Could you check a few things on this model? Use its own coordinates, in mm. Face numbers are marked on the shaded views. A direction names the side the tool comes from. Give positions to 0.01 mm unless a question says otherwise; leave off trailing zeros. Loops run counter-clockwise (first coordinate to the right, second up) from the corner with the lowest first, then second, coordinate; pieces in that order, holes last. Notation, with made-up numbers: (-23.75, 15.25) - (1.25, 15.25) arc R26 cw to (1.25, 35.25) - close; hole circle Ø8 at (13, 47.25). An arc over 180 degrees is marked (long way). Write each question's results on one line, items separated by ' | '. Start each with the question number.
1) I want a section at B-B, the plane x = -5. Write out the boundary of the cut face in (y, z), and give its area (3 significant figures).
2) I want a section at C-C, the plane z = 2.25. Write out the boundary of the cut face in (x, y).
3) I want a section at D-D, the plane y = -4.25. Write out the boundary of the cut face in (x, z).
4) I'm going to push flat-ended pins straight in: pin 1 (3.5 mm diameter, centred on x = -8, y = -2, fed in from +Z); pin 2 (1.8 mm diameter, centred on y = -5.5, z = 2.5, fed in from +X); pin 3 (0.7 mm diameter, centred on x = -8, z = 1.5, fed in from +Y); pin 4 (1.1 mm diameter, centred on x = -7.5, z = 1.5, fed in from -Y). Where does each tip first touch, or does it pass through?
5) On a 3-axis mill with a long thin cutter (end or side, diameter ignored), from which of +Z, -Z, +X, -X, +Y, -Y can I reach the whole of each face in a straight line? I mean the marked faces 1, 2 and 3. Say none if no direction works.
6) If I drill on probe 1 along Y at (x, z) = (-0.25, 4); probe 2 along Y at (x, z) = (-9, 1.25); probe 3 along Z at (x, y) = (10, 1.5), over which ranges is the centre line in solid material (lowest first)? Write a range as [from, to].
7) I want a section at A-A, the plane y = 0. Write out the boundary of the cut face in (x, z).
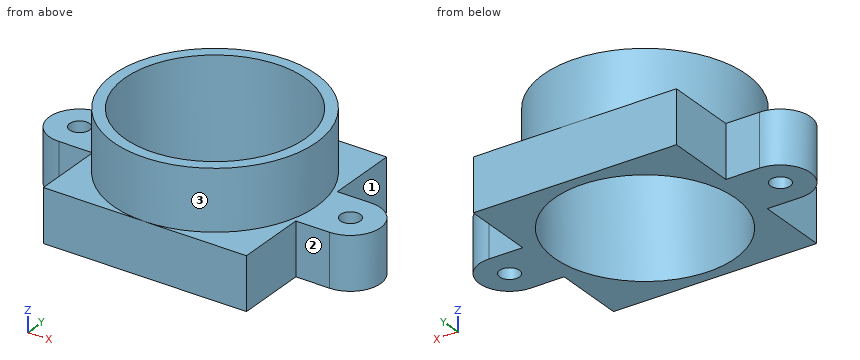
Autodesk Inventor part; units mm, degrees
ref_plane "YZ Plane" through (0, 0, 0) normal (1, 0, 0) x (0, 1, 0)
ref_plane "XZ Plane" through (0, 0, 0) normal (0, 1, 0) x (-1, 0, 0)
ref_plane "XY Plane" through (0, 0, 0) normal (0, 0, 1) x (1, 0, 0)
sketch "Skizze1" plane through (0, 0, 0) normal (0, 0, 1) x (1, 0, 0)
  line L0 (-6.75, -6.75) -> (6.75, -6.75)
  line L1 (6.75, 6.75) -> (-6.75, 6.75)
  line L2 (-6.75, -6.75) -> (6.75, 6.75) construction
  line L3 (6.75, -6.75) -> (-6.75, 6.75) construction
  line L4 (-6.75, 2) -> (-9, 2)
  line L5 (-9, -2) -> (-6.75, -2)
  line L6 (6.75, 2) -> (9, 2)
  line L7 (9, -2) -> (6.75, -2)
  arc A0 (-9, 2) -> (-9, -2) centre (-9, 0) ccw
  arc A1 (9, -2) -> (9, 2) centre (9, 0) ccw
  line L8 (-6.75, 6.75) -> (-6.75, 2)
  line L9 (-6.75, -2) -> (-6.75, -6.75)
  line L10 (6.75, -6.75) -> (6.75, -2)
  line L11 (6.75, 2) -> (6.75, 6.75)
  line L12 (0, 9.45) -> (0, -9.45)
  line L13 (-15.4, 0) -> (15.4, 0)
  point P0 (0, 0)
  dimension "d0" = 13.5
  dimension "d1" = 13.5
  dimension "d2" = 18
  dimension "d3" = 4
extrude "Extrusion1" add sketch "Skizze1" along normal blind 3.5
sketch "Skizze4" plane through (0, 0, 3.5) normal (0, 0, 1) x (1, 0, 0)
  arc A0 (-9, 2) -> (-9, -2) centre (-9, 0) ccw
  arc A1 (9, -2) -> (9, 2) centre (9, 0) ccw
  point P0 (0, 0)
hole "Bohrung1" at (-9, 0, 3.5) at (9, 0, 3.5) direction (0, 0, -1) diameter 1.321 end through all
sketch "Skizze2" plane through (0, 0, 3.5) normal (0, 0, 1) x (1, 0, 0)
  circle A0 centre (0, 0) radius 6.75
  circle A1 centre (0, 0) radius 6
  dimension "d6" = 13.5
  dimension "d7" = 12
extrude "Extrusion2" add sketch "Skizze2" along normal blind 4
thread "Gewinde1"
sketch "Skizze3" plane through (0, 0, 3.5) normal (0, 0, 1) x (1, 0, 0)
  circle A0 centre (0, 0) radius 6
extrude "Extrusion3" cut sketch "Skizze3" against normal through all
properties part number "Linsenhalter M12" material "PC/ABS-Kunststoff"
Answers:
1) outline: (-6.75, 0) - (-3.32, 0) - (-3.32, 7.5) - (-4.53, 7.5) - (-4.53, 3.5) - (-6.75, 3.5) - close; (3.32, 0) - (6.75, 0) - (6.75, 3.5) - (4.53, 3.5) - (4.53, 7.5) - (3.32, 7.5) - close | area: 33.8 mm2
2) outline: (-9, -2) - (-6.75, -2) - (-6.75, -6.75) - (6.75, -6.75) - (6.75, -2) - (9, -2) arc R2 ccw to (9, 2) - (6.75, 2) - (6.75, 6.75) - (-6.75, 6.75) - (-6.75, 2) - (-9, 2) arc R2 ccw to start; hole circle Ø1.32 at (-9, 0); hole circle Ø12 at (0, 0); hole circle Ø1.32 at (9, 0)
3) outline: (-6.75, 0) - (-4.24, 0) - (-4.24, 7.5) - (-5.24, 7.5) - (-5.24, 3.5) - (-6.75, 3.5) - close; (4.24, 0) - (6.75, 0) - (6.75, 3.5) - (5.24, 3.5) - (5.24, 7.5) - (4.24, 7.5) - close
4) pin 1: stops at z = 7.5 | pin 2: stops at x = 6.75 | pin 3: stops at y = 2 | pin 4: stops at y = -2
5) face 1: +Z, -Z, +X, +Y | face 2: +Z, -Z, +X, -Y | face 3: +Z
6) probe 1: y = [-6.75, -5.99], [5.99, 6.75] | probe 2: y = [-2, -0.66], [0.66, 2] | probe 3: z = [0, 3.5]
7) outline: (-11, 0) - (-9.66, 0) - (-9.66, 3.5) - (-11, 3.5) - close; (-8.34, 0) - (-6, 0) - (-6, 7.5) - (-6.75, 7.5) - (-6.75, 3.5) - (-8.34, 3.5) - close; (6, 0) - (8.34, 0) - (8.34, 3.5) - (6.75, 3.5) - (6.75, 7.5) - (6, 7.5) - close; (9.66, 0) - (11, 0) - (11, 3.5) - (9.66, 3.5) - close
